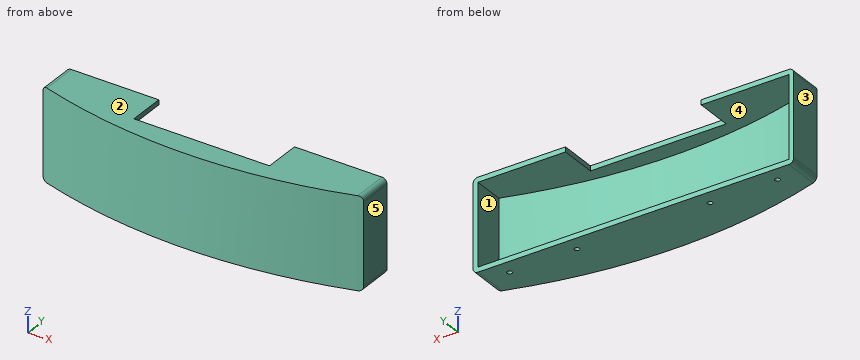
from build123d import *

# Parameters (mm, degrees)
BOSS_EXTRUDE1_DEPTH = 37.24
SHELL1_T            = -2
SKETCH2_W           = 55
SKETCH2_H           = 15
CUT_EXTRUDE1_DEPTH  = 10
SKETCH3_R           = 1
CUT_EXTRUDE2_DEPTH  = 12
FILLET1_R           = 2


with BuildPart() as part:
    # Sketch1 → Boss-Extrude1 (new body)
    with BuildSketch(Plane.XY):
        with BuildLine():
            Line((65, 0), (-65, 0))
            Line((-65, 0), (-65, -14))
            ThreePointArc((-65, -14), (0, -24.210505724), (65, -14))
            Line((65, -14), (65, 0))
        make_face()
    extrude(amount=-BOSS_EXTRUDE1_DEPTH)

    # Shell1
    shell1_openings = [part.faces().sort_by_distance(p)[0] for p in [
        (0, 0, -18.62),
    ]]
    offset(amount=SHELL1_T, openings=shell1_openings, kind=Kind.INTERSECTION)

    # Sketch2 → Cut-Extrude1 (cut)
    with BuildSketch(Plane.XY):
        with Locations((0, -7.5)):
            Rectangle(SKETCH2_W, SKETCH2_H)
    extrude(amount=-CUT_EXTRUDE1_DEPTH, mode=Mode.SUBTRACT)

    # Sketch3 → Cut-Extrude2 (cut)
    with BuildSketch(Plane(origin=(0, 0, -37.24), x_dir=(-1, 0, 0), z_dir=(0, 0, -1))):
        with Locations((-54.285626074, -6.1)):
            Circle(SKETCH3_R)
        with Locations((-26.985626074, -6.1)):
            Circle(SKETCH3_R)
        with Locations((54.285626074, -6.1)):
            Circle(SKETCH3_R)
        with Locations((26.985626074, -6.1)):
            Circle(SKETCH3_R)
    extrude(amount=-CUT_EXTRUDE2_DEPTH, mode=Mode.SUBTRACT)

    # Fillet1
    fillet1_edges = [part.edges().sort_by_distance(p)[0] for p in [
        (65, -7, -37.24),
        (-65, -7, -37.24),
        (65, -7, 0),
        (-65, -7, 0),
    ]]
    fillet(fillet1_edges, radius=FILLET1_R)


solid = part.part
Could you check a few things on this model? Use its own coordinates, in mm. Face numbers are marked on the shaded views. A direction names the side the tool comes from. Round coordinates to 2 decimals unless told otherwise and drop trailing zeros. Order: outer loops, then holes, each group sorted by start corner. A loop starts at its lowest first (then second) coordinate and runs counter-clockwise, first axis right, second up.
(1) If we mould it in two halves opening along Z, with no side actions, what happens to the marked faces 1, 2 and 3? For each: released by +Z, released by -Z, zero draft, split by the parting line, or undercut.
Response values:
face 1: undercut
face 2: released by +Z
face 3: zero draft
(2) Imagine slicing it at A-A (y = -1.75). Write out the boundary of the cut face in (x, z), plus the area to 3 significant figures.
Response values:
outline: (-65, -35.24) arc R2 ccw to (-63, -37.24) - (63, -37.24) arc R2 ccw to (65, -35.24) - (65, -2) arc R2 ccw to (63, 0) - (27.5, 0) - (27.5, -2) - (63, -2) - (63, -35.24) - (-63, -35.24) - (-63, -2) - (-27.5, -2) - (-27.5, 0) - (-63, 0) arc R2 ccw to (-65, -2) - close
area: 540 mm2
(3) I'm going to push flat-ended pins straight in: pin 1 (4 mm diameter, centred on x = 8, y = -7.5, fed in from +Z); pin 2 (1 mm diameter, centred on y = -4, z = -1.5, fed in from +X); pin 3 (1 mm diameter, centred on x = -2, z = -1.5, fed in from +Y); pin 4 (1.2 mm diameter, centred on x = -26.99, y = -6.1, fed in from -Z). Where does each tip first touch, or does it pass through?
Response values:
pin 1: stops at z = -35.24
pin 2: stops at x = 65
pin 3: stops at y = -15
pin 4: stops at z = -2
(4) Imagine slicing it at C-C (x = -6). Write out the boundary of the cut face in (y, z), plus the area to 3 significant figures.
Response values:
outline: (-24.13, -37.24) - (0, -37.24) - (0, -35.24) - (-22.12, -35.24) - (-22.12, -2) - (-15, -2) - (-15, 0) - (-24.13, 0) - close
area: 133 mm2
(5) Please list where these lines run through material, in increasing order: line 1 along Z through (x, y) = (-52, -4.75); line 2 along X through (y, z) = (-9, -14.5); line 3 along Z through (x, y) = (-1, -1.25).
Response values:
line 1: z = -37.24 to -35.24, -2 to 0
line 2: x = -65 to -63, 63 to 65
line 3: z = -37.24 to -35.24
(6) Which directions (+Z, -Z, +X, -X, +Y, -Y) give clear straight access to the entire face, cutting with the end or side of a thin tool? Please do the marked faces 4 and 5.
Response values:
face 4: +Y
face 5: +Z, -Z, +X, +Y, -Y
(7) Imagine slicing it at B-B (z = -22.5). Write out the boundary of the cut face in (x, y).
Response values:
outline: (-65, -14) arc R212 ccw to (65, -14) - (65, 0) - (63, 0) - (63, -12.54) arc R210 cw to (-63, -12.54) - (-63, 0) - (-65, 0) - close
